```python
from build123d import *

# Parameters (mm, degrees)
BOSS_EXTRUDE1_DEPTH      = 4.7625
BOSS_EXTRUDE2_DEPTH      = 41.275
BOSS_EXTRUDE4_START      = 41.275
BOSS_EXTRUDE4_DEPTH      = 4.7625
BOSS_EXTRUDE5_START      = -41.275
BOSS_EXTRUDE5_DEPTH      = 4.7625
BOSS_EXTRUDE3_DEPTH      = 4.7625
CUT_EXTRUDE1_DEPTH       = 197.1201289744139
FILLET3_R                = 4.7625
FILLET5_R                = 29.209999999999997
F_1_4_CLEARANCE_HOLE1_D  = 6.7564
F_5_16_CLEARANCE_HOLE1_D = 8.4328
F_1_4_CLEARANCE_HOLE2_D  = 7.14248
FILLET6_R                = 2.3812499999999996


with BuildPart() as part:
    # Sketch1 → Boss-Extrude1 (new body)
    with BuildSketch(Plane(origin=(0, 0, 0), x_dir=(1, 0, 0), z_dir=(0, 1, 0))):
        Polygon((41.275, -25.39999999999999), (-41.275, -25.400000000000002), (-41.275, 25.4), (-16.510000000000005, 25.4), (-16.509999999999998, -3.1750000000000003), (16.509999999999998, -3.1749999999999963), (16.509999999999998, 25.400000000000002), (41.275, 25.400000000000006), align=None)
    extrude(amount=BOSS_EXTRUDE1_DEPTH)

    # Sketch6 → Boss-Extrude2 (add, symmetric)
    with BuildSketch(Plane(origin=(0, 0, 0), x_dir=(0, 0, -1), z_dir=(1, 0, 0))):
        Polygon((-22.20613588199718, 0), (-47.01090584437518, -60.46162678329637), (-59.41727262806233, -67.62444598552347), (-61.79852262806233, -63.50000000000006), (-50.8, -57.15), (-25.39999999999999, 4.7625), (-25.39999999999999, 0), align=None)
    extrude(amount=BOSS_EXTRUDE2_DEPTH, both=True)

    # Sketch10 → Boss-Extrude4 (add)
    with BuildSketch(Plane(origin=(0, 0, 0), x_dir=(0, 0, -1), z_dir=(1, 0, 0)).offset(BOSS_EXTRUDE4_START)):
        Polygon((-17.05842561014821, 0), (-43.22181168875039, -63.77325356659284), (-79.03306788418706, -84.44889197104685), (-81.41431788418706, -80.32444598552347), (-47.01090584437518, -60.46162678329637), (-22.20613588199718, 0), align=None)
    extrude(amount=-BOSS_EXTRUDE4_DEPTH)

    # Sketch10<2> → Boss-Extrude5 (add)
    with BuildSketch(Plane(origin=(0, 0, 0), x_dir=(0, 0, -1), z_dir=(1, 0, 0)).offset(BOSS_EXTRUDE5_START)):
        Polygon((-17.05842561014821, 0), (-43.22181168875039, -63.77325356659284), (-79.03306788418706, -84.44889197104685), (-81.41431788418706, -80.32444598552347), (-47.01090584437518, -60.46162678329637), (-22.20613588199718, 0), align=None)
    extrude(amount=BOSS_EXTRUDE5_DEPTH)

    # Sketch7 → Boss-Extrude3 (add)
    with BuildSketch(Plane(origin=(0, -20.865454743874867, -12.046675913140254), x_dir=(1, 0, 0), z_dir=(0, 0.866025403784436, 0.5000000000000046))):
        with BuildLine():
            Line((-87.3125, -167.81909051224963), (-87.31250000000001, -97.96909051224961))
            ThreePointArc((-87.31250000000001, -97.96909051224961), (-84.50480271700945, -89.35923141913764), (-77.16122665481106, -84.05972877692089))
            Line((-77.16122665481106, -84.05972877692089), (-41.275, -72.5690905122496))
            Line((-41.275, -72.5690905122496), (41.275, -72.5690905122496))
            Line((41.275, -72.5690905122496), (77.16122665481105, -84.0597287769209))
            ThreePointArc((77.16122665481105, -84.0597287769209), (84.50480271700943, -89.35923141913766), (87.31250000000001, -97.96909051224961))
            Line((87.31250000000001, -97.96909051224961), (87.31250000000001, -167.81909051224963))
            ThreePointArc((87.31250000000001, -167.81909051224963), (80.4839803351822, -180.18162983863905), (66.38372511516263, -180.98404004522925))
            Line((66.38372511516263, -180.98404004522925), (0, -149.09666116895025))
            Line((0, -149.09666116895025), (-66.38372511516263, -180.98404004522925))
            ThreePointArc((-66.38372511516263, -180.98404004522925), (-80.48398033518218, -180.18162983863903), (-87.3125, -167.81909051224963))
        make_face()
    extrude(amount=-BOSS_EXTRUDE3_DEPTH)

    # Sketch11 → Cut-Extrude1 (cut, through all)
    with BuildSketch(Plane(origin=(0, 9.605402363534044, 23.413168261114233), x_dir=(1, 0, 0), z_dir=(0, 0.37955635625630607, 0.9251686183747458))):
        Polygon((-25.400000388402205, -59.45484943793708), (-9.52500014565082, -43.57984943793708), (-8.657059559184285, -43.57984943793708), (-1.1112499999999998, -51.12565911250755), (-1.1112499999999998, -59.45484943793708), align=None)
        Polygon((1.1112499999999998, -59.45484943793708), (25.399999611597792, -59.45484943793708), (9.524999854349167, -43.57984943793708), (8.657059789956651, -43.57984943793708), (1.1112499999999998, -51.12565911250755), align=None)
        Polygon((0.4339700458708439, -48.65984943793709), (7.519485019617413, -41.57433457253814), (0, -34.05484943793708), (-7.519485012578843, -41.574334335532285), (-0.43397001852167266, -48.65984943793709), align=None)
    extrude(amount=-CUT_EXTRUDE1_DEPTH, mode=Mode.SUBTRACT)

    # Fillet3
    fillet3_edges = [part.edges().sort_by_distance(p)[0] for p in [
        (-41.275, 2.38125, -25.4),
    ]]
    fillet(fillet3_edges, radius=FILLET3_R)
    fillet3_2_edges = [part.edges().sort_by_distance(p)[0] for p in [
        (-41.275, -59.21222299276168, 49.60937499999998),
    ]]
    fillet(fillet3_2_edges, radius=FILLET3_R)
    fillet3_3_edges = [part.edges().sort_by_distance(p)[0] for p in [
        (-16.510000000000005, 2.38125, -25.4),
    ]]
    fillet(fillet3_3_edges, radius=FILLET3_R)
    fillet3_4_edges = [part.edges().sort_by_distance(p)[0] for p in [
        (-38.89375, 0, 17.05842561014821),
    ]]
    fillet(fillet3_4_edges, radius=FILLET3_R)
    fillet3_5_edges = [part.edges().sort_by_distance(p)[0] for p in [
        (0, 0, 22.20613588199718),
    ]]
    fillet(fillet3_5_edges, radius=FILLET3_R)
    fillet3_6_edges = [part.edges().sort_by_distance(p)[0] for p in [
        (38.89375, 0, 17.05842561014821),
    ]]
    fillet(fillet3_6_edges, radius=FILLET3_R)
    fillet3_7_edges = [part.edges().sort_by_distance(p)[0] for p in [
        (-38.89375, -63.77325356659284, 43.22181168875039),
    ]]
    fillet(fillet3_7_edges, radius=FILLET3_R)
    fillet3_8_edges = [part.edges().sort_by_distance(p)[0] for p in [
        (0, -60.46162678329637, 47.01090584437518),
    ]]
    fillet(fillet3_8_edges, radius=FILLET3_R)
    fillet3_9_edges = [part.edges().sort_by_distance(p)[0] for p in [
        (-0.7533233620346138, -57.15, 50.8),
    ]]
    fillet(fillet3_9_edges, radius=FILLET3_R)
    fillet3_10_edges = [part.edges().sort_by_distance(p)[0] for p in [
        (0, 4.7625, 25.4),
    ]]
    fillet(fillet3_10_edges, radius=FILLET3_R)
    fillet3_11_edges = [part.edges().sort_by_distance(p)[0] for p in [
        (-16.509999999999998, 2.38125, 3.1750000000000003),
    ]]
    fillet(fillet3_11_edges, radius=FILLET3_R)
    fillet3_12_edges = [part.edges().sort_by_distance(p)[0] for p in [
        (16.509999999999998, 2.38125, 3.1749999999999963),
    ]]
    fillet(fillet3_12_edges, radius=FILLET3_R)
    fillet3_13_edges = [part.edges().sort_by_distance(p)[0] for p in [
        (16.509999999999998, 2.38125, -25.400000000000002),
    ]]
    fillet(fillet3_13_edges, radius=FILLET3_R)
    fillet3_14_edges = [part.edges().sort_by_distance(p)[0] for p in [
        (38.89375, -63.77325356659284, 43.22181168875039),
    ]]
    fillet(fillet3_14_edges, radius=FILLET3_R)
    fillet3_15_edges = [part.edges().sort_by_distance(p)[0] for p in [
        (41.275, 2.38125, -25.400000000000006),
    ]]
    fillet(fillet3_15_edges, radius=FILLET3_R)
    fillet3_16_edges = [part.edges().sort_by_distance(p)[0] for p in [
        (41.275, -59.0883646148863, 49.68088466780772),
    ]]
    fillet(fillet3_16_edges, radius=FILLET3_R)

    # Fillet5
    fillet5_edges = [part.edges().sort_by_distance(p)[0] for p in [
        (0, -97.47600832111236, 115.88419527861113),
    ]]
    fillet(fillet5_edges, radius=FILLET5_R)

    # 1/4 Clearance Hole1 (through all)
    with Locations(Plane(origin=(0, 4.7625, 0), x_dir=(1, 0, 0), z_dir=(0, 1, 0))):
        with Locations((-31.75, -15.875), (31.75, -15.875)):
            Hole(F_1_4_CLEARANCE_HOLE1_D / 2)

    # 5/16 Clearance Hole1 (through all)
    with Locations(Plane(origin=(0, 4.7625, 0), x_dir=(1, 0, 0), z_dir=(0, 1, 0))):
        with Locations((-26.19375, 9.525), (26.19375, 9.525)):
            Hole(F_5_16_CLEARANCE_HOLE1_D / 2)

    # 1/4 Clearance Hole2 (through all)
    with Locations(Plane(origin=(0, -20.865454743874867, -12.046675913140254), x_dir=(1, 0, 0), z_dir=(0, 0.866025403784436, 0.5000000000000046))):
        with Locations((-72.7075, -97.969090512), (-72.7075, -167.819090512), (72.7075, -167.819090512), (72.7075, -97.969090512)):
            Hole(F_1_4_CLEARANCE_HOLE2_D / 2)

    # Fillet6
    fillet6_edges = [part.edges().sort_by_distance(p)[0] for p in [
        (38.89375, -84.44889197104685, 79.03306788418706),
        (-38.89375, -84.44889197104685, 79.03306788418706),
    ]]
    fillet(fillet6_edges, radius=FILLET6_R)


solid = part.part
```
Geometry: final body of the model. Coordinates: model frame, mm. A direction names the side the tool comes from. Round coordinates to 2 decimals unless told otherwise and drop trailing zeros. Loops run counter-clockwise (first coordinate to the right, second up) from the corner with the lowest first, then second, coordinate; pieces in that order, holes last. Notation, with made-up numbers: (36.25, 46.25) -> (46.25, 46.25) arc R17 ccw to (46.25, 61.25) -> close; hole circle Ø11 at (55.25, 84). An arc over 180 degrees is marked (long way). Use one line per item in the form item = value.
Item 1: Draft query along Y for faces 4 (the cylindrical face through (-42.166, -58.46, 49.233)), 5 (the flat face through (3.81, -26.32, 35.61)), 6 (the flat face through (39.892, -107.028, 132.496)), 7 (the cylindrical face through (15.078, 2.415, 1.817)). Return one class per face: released by +Y, released by -Y, zero draft, split by the parting line, or undercut.
Evaluation:
face_4 = released by +Y
face_5 = undercut
face_6 = released by -Y
face_7 = zero draft
Item 2: Material intervals for probe 1 along Y at (x, z) = (-10, 9); probe 2 along X at (y, z) = (-8, 28) (3 decimals); probe 3 along Z at (x, y) = (-31.75, 3.75), sorted ascending.
Evaluation:
probe_1 = 0 to 4.76
probe_2 = -41.275 to 41.275
probe_3 = -25.4 to 12.5, 19.25 to 25.14
Item 3: Contact query for flat-ended pins moving along their axis: pin 1 Ø7.5 at (x, z) = (-26.19, -9.52) entering from -Y; pin 2 Ø8 at (x, y) = (-17.5, -21) entering from -Z; pin 3 Ø12 at (x, y) = (9, -13.5) entering from -Z; pin 4 Ø8.5 at (y, z) = (-42, 42) entering from -X (3 decimals). Output: stop coordinate, or through.
Evaluation:
pin_1 = through
pin_2 = 29.18
pin_3 = 25.28
pin_4 = -41.275
Item 4: Cut plane A-A on z = 6. Output: boundary loops of the cut face in (x, y) (1 decimal), then the cut area to 3 significant figures.
Evaluation:
outline = (-41.3, 0) -> (41.3, 0) -> (41.3, 4.8) -> (-41.3, 4.8) -> close
area = 393 mm2
Item 5: Access query for faces 1 (the flat face through (0, 2, 3.175)), 2 (the cylindrical face through (0.183, -99.103, 118.635)), 3 (the cylindrical face through (0.511, -0.785, 21.632)). Directions: +Z, -Z, +X, -X, +Y, -Y. A direction counts if a zero-diameter tool reaches every point of the face in a straight line with its end or side. Return the directions, or none.
Evaluation:
face_1 = -Z, +Y, -Y
face_2 = +Z, -Y
face_3 = -Z, -Y
Item 6: Cut plane B-B on x = 56. Output: boundary loops of the cut face in (y, z), then the cut area to 3 significant figures.
Evaluation:
outline = (-112.99, 137.99) -> (-63.63, 52.5) -> (-59.51, 54.88) -> (-108.86, 140.37) -> close
area = 470 mm2
